Design review of the part shown in the three views and the two pictorial views. Dimensions are in mm from the part's minimum x, y and z. A direction names the side the tool comes from. Give positions to 0.01 mm unless a question says otherwise; leave off trailing zeros. Loops run counter-clockwise (first coordinate to the right, second up) from the corner with the lowest first, then second, coordinate; pieces in that order, holes last. Notation, with made-up numbers: (66, -38) -> (71, -38) arc R14 cw to (71, -26) -> close; hole circle Ø3 at (-23, 18). An arc over 180 degrees is marked (long way). One line per question, with ' | ' between items. Start each with the question number.
(1) Consider section C-C (z = 169). Write out the cut boundary in (x, y), and give its area (3 significant figures).
(2) Tool access review of the marked faces 1, 2 and 3: name each direction out of +Z, -Z, +X, -X, +Y, -Y from which nothing blocks a thin tool from reaching the whole face with its end or side.
(3) Wall thickness on probe 1 along X at (y, z) = (276.5, 234.5); probe 2 along Z at (x, y) = (596, 154.5); probe 3 along Y at (x, z) = (841.5, 257.5): over which ranges is each line inside the solid? List them lowest first.
(4) Consider section A-A (x = 443). Write out the cut boundary in (y, z).
(5) Insertion check: P1, Ø11.5, axis at y = 18, z = 298, coming from the -X side; P2, Ø4, axis at x = 208, y = 164, coming from the -Z side. Each pin has a flat end and moves straight along its axis. Give the tip position at first contact, or say it passes through.
(6) Consider section B-B (y = 161). Write out the cut boundary in (x, z).
(7) Draft analysis for pull direction Z (two halves, no side actions). For the marked faces 4, 5, 6 and 7, state which applies: +Z half, -Z half, draft (parallel to the pull), parting line (faces both ways), or undercut.
(8) Consider section D-D (x = 190). Write out the cut boundary in (y, z).
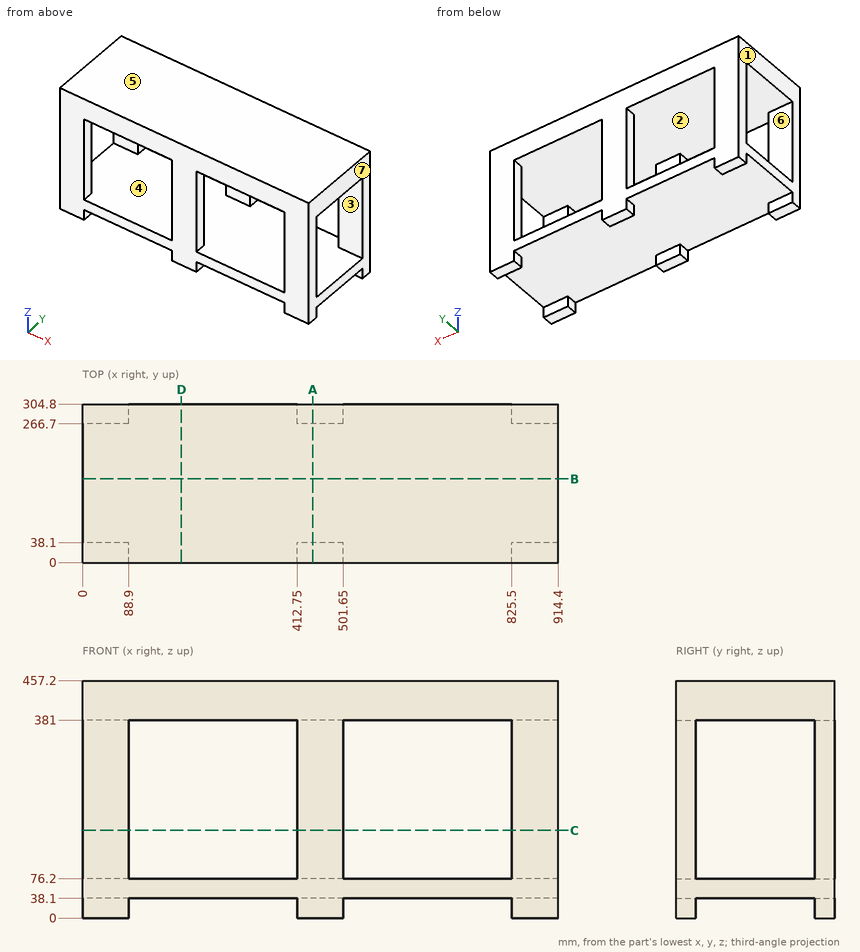
A:
1) outline: (0, 0) -> (88.9, 0) -> (88.9, 38.1) -> (0, 38.1) -> close; (0, 266.7) -> (88.9, 266.7) -> (88.9, 304.8) -> (0, 304.8) -> close; (412.75, 0) -> (501.65, 0) -> (501.65, 38.1) -> (412.75, 38.1) -> close; (412.75, 266.7) -> (501.65, 266.7) -> (501.65, 304.8) -> (412.75, 304.8) -> close; (825.5, 0) -> (914.4, 0) -> (914.4, 38.1) -> (825.5, 38.1) -> close; (825.5, 266.7) -> (914.4, 266.7) -> (914.4, 304.8) -> (825.5, 304.8) -> close | area: 20,300 mm^2
2) face 1: +Z, -Z, -X, +Y, -Y | face 2: none | face 3: +X, -X
3) probe 1: x = 0 to 88.9, 412.75 to 501.65, 825.5 to 914.4 | probe 2: z = 38.1 to 76.2, 381 to 457.2 | probe 3: y = 0 to 38.1, 266.7 to 304.8
4) outline: (0, 0) -> (38.1, 0) -> (38.1, 38.1) -> (266.7, 38.1) -> (266.7, 0) -> (304.8, 0) -> (304.8, 457.2) -> (0, 457.2) -> close; hole (38.1, 76.2) -> (266.7, 76.2) -> (266.7, 381) -> (38.1, 381) -> close
5) P1: stops at x = 0 | P2: stops at z = 38.1
6) outline: (0, 38.1) -> (914.4, 38.1) -> (914.4, 76.2) -> (0, 76.2) -> close; (0, 381) -> (914.4, 381) -> (914.4, 457.2) -> (0, 457.2) -> close
7) face 4: undercut | face 5: +Z half | face 6: undercut | face 7: draft
8) outline: (0, 38.1) -> (304.8, 38.1) -> (304.8, 76.2) -> (0, 76.2) -> close; (0, 381) -> (304.8, 381) -> (304.8, 457.2) -> (0, 457.2) -> close
